Design review of the part built by this model. Coordinates are the model's own, in mm. Give positions to 0.01 mm unless a question says otherwise; leave off trailing zeros. Write each loop counter-clockwise with the first axis right and the second up, starting at its lowest first coordinate (ties: lowest second). Pieces come first, ordered by that corner, then holes.
```python
from build123d import *

# Parameters (mm, degrees)
CROQUIS1_W              = 50
CROQUIS1_H              = 20
SALIENTE_EXTRUIR1_DEPTH = 5


with BuildPart() as part:
    # Croquis1 → Saliente-Extruir1 (new body)
    with BuildSketch(Plane(origin=(0, 0, 0), x_dir=(1, 0, 0), z_dir=(0, 1, 0))):
        Rectangle(CROQUIS1_W, CROQUIS1_H)
        Polygon((25, 10), (50, 2), (50, 0), (50, -2), (25, -10), align=None)
    extrude(amount=SALIENTE_EXTRUIR1_DEPTH)


solid = part.part
```
(1) Consider section B-B, the plane x = 37. Give the boundary of the cut face in (y, z), then the cut area to 3 significant figures.
Resolved:
outline: (0, -6.16) - (5, -6.16) - (5, 6.16) - (0, 6.16) - close
area: 61.6 mm2
(2) Consider section A-A, the plane y = 2.1. Give the boundary of the cut face in (x, z).
Resolved:
outline: (-25, -10) - (25, -10) - (50, -2) - (50, 2) - (25, 10) - (-25, 10) - close
(3) To check wall thickness, follow L1, parallel to Z at x = 45, y = 2.1; L2, parallel to Z at x = 28, y = 3.6. State the ranges of each line that lie inside material, in increasing order.
Resolved:
L1: z = -3.6 to 3.6
L2: z = -9.04 to 9.04
(4) Clearance check with a flat-ended pin moving along its axis: P1, Ø1.5, axis at x = 26.5, y = 1, coming from the +Z side. State where the tip first meets the part, or that it passes through.
Resolved:
P1: stops at z = 9.76
(5) Consider section C-C, the plane z = 7.5. Give the boundary of the cut face in (x, y).
Resolved:
outline: (-25, 0) - (32.81, 0) - (32.81, 5) - (-25, 5) - close
